Part model, mm, in its own coordinate system. Face numbers are marked on the shaded views. Round coordinates to 2 decimals unless told otherwise and drop trailing zeros. Loops run counter-clockwise (first coordinate to the right, second up) from the corner with the lowest first, then second, coordinate; pieces in that order, holes last.
(1) Cut at C-C on z = 15.5. List the corners of the cut face in (x, y).
(2) Probe probe 1 along Y at (x, z) = (0, 17.9); probe 2 along X at (y, z) = (-20, 13.5); probe 3 along Z at (x, y) = (-15.5, -20.5). List the from-to ranges inside material, lowest first.
(3) Flat gauge pins, fed straight in: pin 1 (12.5 mm diameter, centred on x = 5.5, y = -15, fed in from -Z); pin 2 (5 mm diameter, centred on x = 0, y = -12.5, fed in from +Z); pin 3 (0.8 mm diameter, centred on y = -16.5, z = 15.5, fed in from +X). Where does each tip first touch, or does it go through?
(4) Cut at A-A on y = -12.5. List the corners of the cut face in (x, z).
(5) Cut at D-D on y = -18. List the corners of the cut face in (x, z).
(6) Mould opens along X. For the marked faces 1, 2 and 3 say: +X half, -X half, draft (parallel to the pull), parting line (faces both ways), or undercut.
(7) Cut at B-B on x = 0. List the corners of the cut face in (y, z), then the cut area to 3 significant figures.
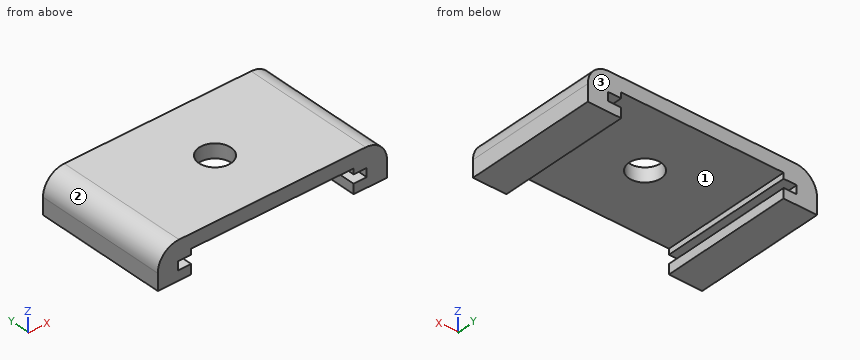
from build123d import *

# Parameters (mm, degrees)
F1_DEPTH = 50
F3_DEPTH = 25
F6_D     = 6


with BuildPart() as f1:
    # F0 (on Front) → F1 (new body)
    with BuildSketch(Plane.XZ):
        with BuildLine():
            Line((-17.75, 14.9), (-17.75, 13.3))
            Line((-17.75, 13.3), (-14.55, 13.3))
            ThreePointArc((-14.55, 13.3), (-13.913604, 13.036396), (-13.65, 12.4))
            Line((-13.65, 12.4), (-13.65, 0.9))
            ThreePointArc((-13.65, 0.9), (-13.386396, 0.263604), (-12.75, 0))
            Line((-12.75, 0), (0, 0))
            Line((0, 0), (12.75, 0))
            ThreePointArc((12.75, 0), (13.386396, 0.263604), (13.65, 0.9))
            Line((13.65, 0.9), (13.65, 12.4))
            ThreePointArc((13.65, 12.4), (13.913604, 13.036396), (14.55, 13.3))
            Line((14.55, 13.3), (17.75, 13.3))
            Line((17.75, 13.3), (17.75, 14.9))
            Line((17.75, 14.9), (13.25, 14.9))
            ThreePointArc((13.25, 14.9), (12.401472, 14.548528), (12.05, 13.7))
            Line((12.05, 13.7), (12.05, 2.5))
            ThreePointArc((12.05, 2.5), (11.786396, 1.863604), (11.15, 1.6))
            Line((11.15, 1.6), (0, 1.6))
            Line((0, 1.6), (-11.15, 1.6))
            ThreePointArc((-11.15, 1.6), (-11.786396, 1.863604), (-12.05, 2.5))
            Line((-12.05, 2.5), (-12.05, 13.7))
            ThreePointArc((-12.05, 13.7), (-12.401472, 14.548528), (-13.25, 14.9))
            Line((-13.25, 14.9), (-17.75, 14.9))
        make_face()
    extrude(amount=F1_DEPTH)


with BuildPart() as f3:
    # F2 (on Front) → F3 (new body)
    with BuildSketch(Plane.XZ):
        with BuildLine():
            Line((-21.562627, 11.464062), (-15.28198, 11.464062))
            Line((-15.28198, 11.464062), (-15.28198, 15.950238))
            Line((-15.28198, 15.950238), (0, 15.950238))
            Line((0, 15.950238), (15.28198, 15.950238))
            Line((15.28198, 15.950238), (15.28198, 11.464062))
            Line((15.28198, 11.464062), (21.562627, 11.464062))
            Line((21.562627, 11.464062), (21.562627, 14.577311))
            ThreePointArc((21.562627, 14.577311), (20.391054, 17.405738), (17.562627, 18.577311))
            Line((17.562627, 18.577311), (0, 18.577311))
            Line((0, 18.577311), (-17.562627, 18.577311))
            ThreePointArc((-17.562627, 18.577311), (-20.391054, 17.405738), (-21.562627, 14.577311))
            Line((-21.562627, 14.577311), (-21.562627, 11.464062))
        make_face()
    extrude(amount=F3_DEPTH)

    # F4: cut F1
    add(f1.part, mode=Mode.SUBTRACT)

    # F6 (through all)
    with Locations(Plane.XY.offset(18.577311)):
        with Locations((0, -12.5)):
            Hole(F6_D / 2)


solid = f3.part
Final values:
1. outline: (-21.45, -25) - (-15.28, -25) - (-15.28, 0) - (-21.45, 0) - close; (15.28, -25) - (21.45, -25) - (21.45, 0) - (15.28, 0) - close
2. probe 1: y = -25 to -15.5, -9.5 to 0
2. probe 2: x = -21.56 to -17.75, 17.75 to 21.56
2. probe 3: z = 11.46 to 13.3, 14.9 to 18.58
3. pin 1: stops at z = 15.95
3. pin 2: passes through
3. pin 3: stops at x = 21.53
4. outline: (-21.56, 11.46) - (-15.28, 11.46) - (-15.28, 13.3) - (-17.75, 13.3) - (-17.75, 14.9) - (-15.28, 14.9) - (-15.28, 15.95) - (-3, 15.95) - (-3, 18.58) - (-17.56, 18.58) arc R4 ccw to (-21.56, 14.58) - close; (3, 15.95) - (15.28, 15.95) - (15.28, 14.9) - (17.75, 14.9) - (17.75, 13.3) - (15.28, 13.3) - (15.28, 11.46) - (21.56, 11.46) - (21.56, 14.58) arc R4 ccw to (17.56, 18.58) - (3, 18.58) - close
5. outline: (-21.56, 11.46) - (-15.28, 11.46) - (-15.28, 13.3) - (-17.75, 13.3) - (-17.75, 14.9) - (-15.28, 14.9) - (-15.28, 15.95) - (15.28, 15.95) - (15.28, 14.9) - (17.75, 14.9) - (17.75, 13.3) - (15.28, 13.3) - (15.28, 11.46) - (21.56, 11.46) - (21.56, 14.58) arc R4 ccw to (17.56, 18.58) - (-17.56, 18.58) arc R4 ccw to (-21.56, 14.58) - close
6. face 1: undercut
6. face 2: -X half
6. face 3: draft
7. outline: (-25, 15.95) - (-15.5, 15.95) - (-15.5, 18.58) - (-25, 18.58) - close; (-9.5, 15.95) - (0, 15.95) - (0, 18.58) - (-9.5, 18.58) - close
7. area: 49.9 mm2
